```python
from build123d import *

# Parameters (mm, degrees)
ESBO_O1_W                = 60
ESBO_O1_H                = 46
RESSALTO_EXTRUS_O1_DEPTH = 20
ESBO_O2_W                = 26
ESBO_O2_H                = 46
CORTE_EXTRUS_O1_DEPTH    = 16
ESBO_O5_R                = 1.5
CORTE_EXTRUS_O3_DEPTH    = 5
ESBO_O8_R                = 2.5
CORTE_EXTRUS_O5_DEPTH    = 21
ESBO_O9_R                = 5
CORTE_EXTRUS_O6_DEPTH    = 7


with BuildPart() as part:
    # Esboço1 → Ressalto-extrusão1 (new body)
    with BuildSketch(Plane.XY):
        Rectangle(ESBO_O1_W, ESBO_O1_H)
    extrude(amount=RESSALTO_EXTRUS_O1_DEPTH)

    # Esboço2 → Corte-extrusão1 (cut)
    with BuildSketch(Plane.XY.offset(20)):
        with Locations((17, 0)):
            Rectangle(ESBO_O2_W, ESBO_O2_H)
    extrude(amount=-CORTE_EXTRUS_O1_DEPTH, mode=Mode.SUBTRACT)

    # Esboço5 → Corte-extrusão3 (cut, through all)
    with BuildSketch(Plane.XY.offset(4)):
        with Locations((13, 9)):
            Circle(ESBO_O5_R)
        with Locations((13, -8)):
            Circle(ESBO_O5_R)
        with Locations((27, 17)):
            Circle(ESBO_O5_R)
    extrude(amount=-CORTE_EXTRUS_O3_DEPTH, mode=Mode.SUBTRACT)

    # Esboço8 → Corte-extrusão5 (cut, through all)
    with BuildSketch(Plane.XY.offset(20)):
        with Locations((-12, -14)):
            Circle(ESBO_O8_R)
        with Locations((-12, 14)):
            Circle(ESBO_O8_R)
    extrude(amount=-CORTE_EXTRUS_O5_DEPTH, mode=Mode.SUBTRACT)

    # Esboço9 → Corte-extrusão6 (cut)
    with BuildSketch(Plane(origin=(0, 0, 0), x_dir=(-1, 0, 0), z_dir=(0, 0, -1))):
        with Locations((12, -14)):
            Circle(ESBO_O9_R)
        with Locations((12, 14.082568483)):
            Circle(ESBO_O9_R)
    extrude(amount=-CORTE_EXTRUS_O6_DEPTH, mode=Mode.SUBTRACT)


solid = part.part
```
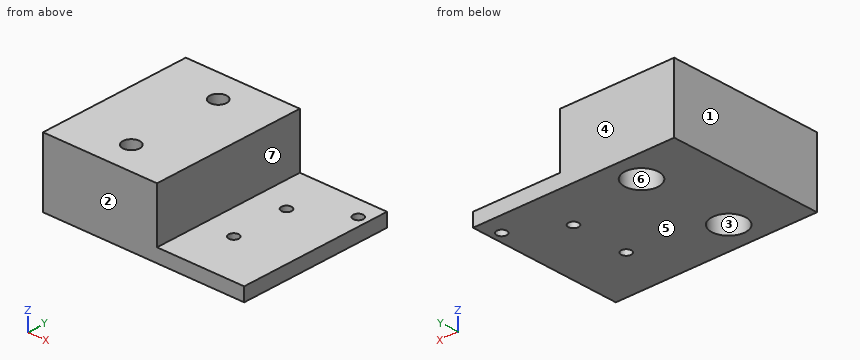
Work out the finished part from the listing and answer in its coordinate system (mm). Face numbers are marked on the shaded views. A direction names the side the tool comes from. Give positions to 0.01 mm unless a question says otherwise; leave off trailing zeros. Loops run counter-clockwise (first coordinate to the right, second up) from the corner with the lowest first, then second, coordinate; pieces in that order, holes last. Notation, with made-up numbers: (-13.5, 68) -> (26.5, 68) arc R30 ccw to (26.5, 97) -> close; hole circle Ø10 at (-21.5, 3.5). An arc over 180 degrees is marked (long way). Use CSV: the item, a comma, the result in double quotes.
1. The part is cut by section D-D (z = 15.5). Write down the section's boundary in (x, y), then the cut area to 3 significant figures.
Found:
outline,"(-30, -23) -> (4, -23) -> (4, 23) -> (-30, 23) -> close; hole circle Ø5 at (-12, -14); hole circle Ø5 at (-12, 14)"
area,"1,520 mm^2"
2. The mould has two halves that part along Y. Classify the marked faces 1, 2, 3 and 4: +Y half, -Y half, draft (parallel to the pull), parting line (faces both ways), or undercut.
Found:
face 1,"draft"
face 2,"-Y half"
face 3,"undercut"
face 4,"+Y half"
3. A tool of negligible diameter and unlimited length cuts with its end or side. For the marked faces 5, 6 and 7, from which of +Z, -Z, +X, -X, +Y, -Y can it reach the whole face along a straight path? Write none if from no direction.
Found:
face 5,"-Z, +X, -X, +Y, -Y"
face 6,"-Z"
face 7,"+Z, +X, +Y, -Y"
4. Flat-ended cylindrical pins translate along their axes: pin 1 Ø3 at (x, y) = (-12.5, 12) entering from -Z; pin 2 Ø4 at (x, y) = (27, 17) entering from +Z; pin 3 Ø3 at (x, z) = (6.5, 8.5) entering from -Y; pin 4 Ø5 at (y, z) = (3, 10) entering from +X. Find the tip coordinate at first contact, or state that the pin passes through.
Found:
pin 1,"z = 7"
pin 2,"z = 4"
pin 3,"through"
pin 4,"x = 4"
5. Straight lines are drawn through the part: line 1 (Y direction, x = -12, z = 5.25); line 2 (Y direction, x = -12, z = 17); line 3 (Z direction, x = 18.5, y = -3). For each, find the intervals that lie inside material, in ascending order.
Found:
line 1,"-23 to -19, -9 to 9.08, 19.08 to 23"
line 2,"-23 to -16.5, -11.5 to 11.5, 16.5 to 23"
line 3,"0 to 4"
6. The part is cut by section A-A (x = 13). Write down the section's boundary in (y, z), then the cut area to 3 significant figures.
Found:
outline,"(-23, 0) -> (-9.5, 0) -> (-9.5, 4) -> (-23, 4) -> close; (-6.5, 0) -> (7.5, 0) -> (7.5, 4) -> (-6.5, 4) -> close; (10.5, 0) -> (23, 0) -> (23, 4) -> (10.5, 4) -> close"
area,"160 mm^2"
7. The part is cut by section B-B (y = -8). Write down the section's boundary in (x, z), then the cut area to 3 significant figures.
Found:
outline,"(-30, 0) -> (11.5, 0) -> (11.5, 4) -> (4, 4) -> (4, 20) -> (-30, 20) -> close; (14.5, 0) -> (30, 0) -> (30, 4) -> (14.5, 4) -> close"
area,"772 mm^2"
8. The part is cut by section C-C (x = 27). Write down the section's boundary in (y, z).
Found:
outline,"(-23, 0) -> (15.5, 0) -> (15.5, 4) -> (-23, 4) -> close; (18.5, 0) -> (23, 0) -> (23, 4) -> (18.5, 4) -> close"
